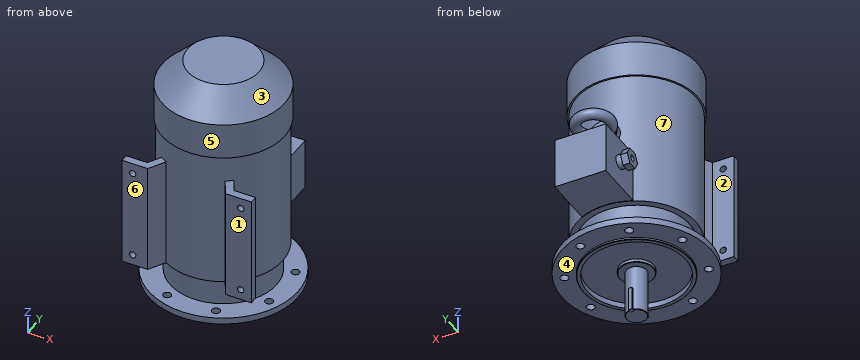
from build123d import *

# Parameters (mm, degrees)
SKETCH_1_R           = 24
EXTRUDE_1_DEPTH      = 110
SKETCH_2_W           = 9
SKETCH_2_H           = 9
EXTRUDE_2_DEPTH      = 0.1
EXTRUDE_2_DEPTH_BACK = 55
SKETCH_3_R           = 175
EXTRUDE_3_DEPTH      = 15
SKETCH_4_R           = 125
SKETCH_4_R_2         = 116
EXTRUDE_4_DEPTH      = 5
SKETCH_5_R           = 116
SKETCH_5_R_2         = 40
CUT_EXTRUDE_1_DEPTH  = 8
CHAMFER_1_SIZE       = 1
SKETCH_6_R           = 9.5
CUT_EXTRUDE_2_DEPTH  = 16
SKETCH_7_R           = 125
EXTRUDE_5_DEPTH      = 68
SKETCH_8_R           = 140
EXTRUDE_6_DEPTH      = 322
SKETCH_9_R           = 144
EXTRUDE_7_DEPTH      = 145
CHAMFER_2_SIZE       = 60
EXTRUDE_8_DEPTH      = 260
CUT_EXTRUDE_3_REACH  = 337
SKETCH_11_R          = 7.5
SKETCH_12_W          = 120
SKETCH_12_H          = 120
EXTRUDE_9_DEPTH      = 245
SKETCH_13_R          = 35
EXTRUDE_10_DEPTH     = 150
CHAMFER_3_SIZE       = 1
SKETCH_15_R          = 12
SKETCH_16_R          = 16
EXTRUDE_11_DEPTH     = 14
EXTRUDE_12_DEPTH     = 16
SKETCH_18_R          = 7
CUT_EXTRUDE_4_DEPTH  = 16


with BuildPart() as part:
    # Эскиз1 → Вытянуть1 (new body)
    with BuildSketch(Plane.XY):
        Circle(SKETCH_1_R)
    extrude(amount=EXTRUDE_1_DEPTH)

    # Эскиз2 → Вытянуть2 (add, two sides)
    with BuildSketch(Plane(origin=(0, 0, 0), x_dir=(-1, 0, 0), z_dir=(0, 0, -1))) as extrude_2_sk:
        with Locations((0, 23)):
            Rectangle(SKETCH_2_W, SKETCH_2_H)
    extrude(amount=EXTRUDE_2_DEPTH)
    extrude(extrude_2_sk.sketch, amount=-EXTRUDE_2_DEPTH_BACK)

    # Эскиз3 → Вытянуть3 (add)
    with BuildSketch(Plane.XY.offset(110)):
        Circle(SKETCH_3_R)
    extrude(amount=EXTRUDE_3_DEPTH)

    # Эскиз4 → Вытянуть4 (add)
    with BuildSketch(Plane(origin=(0, 0, 110), x_dir=(-1, 0, 0), z_dir=(0, 0, -1))):
        with Locations(Location((0, 0, 0), (0, 0, 180))):  # turned: the seam where the file's is
            Circle(SKETCH_4_R)
        Circle(SKETCH_4_R_2, mode=Mode.SUBTRACT)
    extrude(amount=EXTRUDE_4_DEPTH)

    # Эскиз5 → Вырез-Вытянуть1 (cut)
    with BuildSketch(Plane(origin=(0, 0, 110), x_dir=(-1, 0, 0), z_dir=(0, 0, -1))):
        Circle(SKETCH_5_R)
        Circle(SKETCH_5_R_2, mode=Mode.SUBTRACT)
    extrude(amount=-CUT_EXTRUDE_1_DEPTH, mode=Mode.SUBTRACT)

    # Фаска1
    chamfer_1_edges = [part.edges().sort_by_distance(p)[0] for p in [
        (-125, 0, 105),
        (40, 0, 110),
        (-15.297058541, -18.493242009, 0),
    ]]
    chamfer(chamfer_1_edges, length=CHAMFER_1_SIZE)

    # Эскиз6 → Вырез-Вытянуть2 (cut, through all)
    with BuildSketch(Plane(origin=(0, 0, 110), x_dir=(-1, 0, 0), z_dir=(0, 0, -1))):
        with Locations((-57.402514855, 138.581929877)):
            Circle(SKETCH_6_R)
        with Locations((57.402514855, 138.581929877)):
            Circle(SKETCH_6_R)
        with Locations((138.581929877, 57.402514855)):
            Circle(SKETCH_6_R)
        with Locations((138.581929877, -57.402514855)):
            Circle(SKETCH_6_R)
        with Locations((57.402514855, -138.581929877)):
            Circle(SKETCH_6_R)
        with Locations((-57.402514855, -138.581929877)):
            Circle(SKETCH_6_R)
        with Locations((-138.581929877, -57.402514855)):
            Circle(SKETCH_6_R)
        with Locations((-138.581929877, 57.402514855)):
            Circle(SKETCH_6_R)
    extrude(amount=-CUT_EXTRUDE_2_DEPTH, mode=Mode.SUBTRACT)

    # Эскиз7 → Вытянуть5 (add)
    with BuildSketch(Plane.XY.offset(125)):
        Circle(SKETCH_7_R)
    extrude(amount=EXTRUDE_5_DEPTH)

    # Эскиз8 → Вытянуть6 (add)
    with BuildSketch(Plane.XY.offset(193)):
        Circle(SKETCH_8_R)
    extrude(amount=EXTRUDE_6_DEPTH)

    # Эскиз9 → Вытянуть7 (add)
    with BuildSketch(Plane.XY.offset(515)):
        Circle(SKETCH_9_R)
    extrude(amount=EXTRUDE_7_DEPTH)

    # Фаска2
    chamfer_2_edges = [part.edges().sort_by_distance(p)[0] for p in [
        (-144, 0, 660),
    ]]
    chamfer(chamfer_2_edges, length=CHAMFER_2_SIZE)

    # Эскиз10 → Вытянуть8 (add)
    with BuildSketch(Plane(origin=(0, 0, 193), x_dir=(-1, 0, 0), z_dir=(0, 0, -1))):
        Polygon((-152, -160), (-91.607695155, -160), (-51.945448858, -91.302974272), (-67.533906126, -82.302974272), (-102, -142), (-152, -142), align=None)
        Polygon((91.607695155, -160), (51.945448858, -91.302974272), (67.533906126, -82.302974272), (102, -142), (152, -142), (152, -160), align=None)
    extrude(amount=-EXTRUDE_8_DEPTH)

    # Эскиз11 → Вырез-Вытянуть3 (cut, up to next)
    with BuildSketch(Plane.XZ.offset(160), mode=Mode.PRIVATE) as cut_extrude_3_sk1:
        with Locations((-127, 218)):
            Circle(SKETCH_11_R)
    cut_extrude_3_tool1 = extrude(cut_extrude_3_sk1.sketch, amount=-CUT_EXTRUDE_3_REACH, mode=Mode.PRIVATE) & part.part
    add(cut_extrude_3_tool1.solids().sort_by_distance((-127, -160, 218))[0], mode=Mode.SUBTRACT)
    # Эскиз11 → Вырез-Вытянуть3 (cut, up to next)
    with BuildSketch(Plane.XZ.offset(160), mode=Mode.PRIVATE) as cut_extrude_3_sk2:
        with Locations((127, 218)):
            Circle(SKETCH_11_R)
    cut_extrude_3_tool2 = extrude(cut_extrude_3_sk2.sketch, amount=-CUT_EXTRUDE_3_REACH, mode=Mode.PRIVATE) & part.part
    add(cut_extrude_3_tool2.solids().sort_by_distance((127, -160, 218))[0], mode=Mode.SUBTRACT)
    # Эскиз11 → Вырез-Вытянуть3 (cut, up to next)
    with BuildSketch(Plane.XZ.offset(160), mode=Mode.PRIVATE) as cut_extrude_3_sk3:
        with Locations((-127, 428)):
            Circle(SKETCH_11_R)
    cut_extrude_3_tool3 = extrude(cut_extrude_3_sk3.sketch, amount=-CUT_EXTRUDE_3_REACH, mode=Mode.PRIVATE) & part.part
    add(cut_extrude_3_tool3.solids().sort_by_distance((-127, -160, 428))[0], mode=Mode.SUBTRACT)
    # Эскиз11 → Вырез-Вытянуть3 (cut, up to next)
    with BuildSketch(Plane.XZ.offset(160), mode=Mode.PRIVATE) as cut_extrude_3_sk4:
        with Locations((127, 428)):
            Circle(SKETCH_11_R)
    cut_extrude_3_tool4 = extrude(cut_extrude_3_sk4.sketch, amount=-CUT_EXTRUDE_3_REACH, mode=Mode.PRIVATE) & part.part
    add(cut_extrude_3_tool4.solids().sort_by_distance((127, -160, 428))[0], mode=Mode.SUBTRACT)

    # Эскиз12 → Вытянуть9 (add)
    with BuildSketch(Plane(origin=(0, 0, 0), x_dir=(1, 0, 0), z_dir=(0, 1, 0))):
        with Locations((0, -254)):
            Rectangle(SKETCH_12_W, SKETCH_12_H)
    extrude(amount=EXTRUDE_9_DEPTH)

    # Эскиз13 → Вытянуть10 (add)
    with BuildSketch(Plane(origin=(0, 0, 0), x_dir=(1, 0, 0), z_dir=(0, 1, 0))):
        with Locations(Location((0, -371, 0), (0, 0, 90))):  # turned: the seam where the file's is
            Circle(SKETCH_13_R)
    extrude(amount=EXTRUDE_10_DEPTH)

    # Фаска3
    chamfer_3_edges = [part.edges().sort_by_distance(p)[0] for p in [
        (0, 150, 406),
    ]]
    chamfer(chamfer_3_edges, length=CHAMFER_3_SIZE)

    # По траектории1: sweep along a path in Эскиз14
    with BuildLine(Plane.XY.offset(370)) as sweep_1_path:
        CenterArc((0, 188), 38, 0, 360)
    # Эскиз15 → По траектории1 (sweep)
    with BuildSketch(Plane(origin=(0, 0, 0), x_dir=(0, 0, -1), z_dir=(1, 0, 0))):
        with Locations((-370, 226)):
            Circle(SKETCH_15_R)
    sweep(path=sweep_1_path.line)

    # Эскиз16 → Вытянуть11 (add)
    with BuildSketch(Plane.ZY.offset(60)):
        with Locations(Location((254, 185, 0), (0, 0, 180))):  # turned: the seam where the file's is
            Circle(SKETCH_16_R)
    extrude(amount=EXTRUDE_11_DEPTH)

    # Эскиз17 → Вытянуть12 (add)
    with BuildSketch(Plane.ZY.offset(74)):
        Polygon((254, 207.516660498), (234.5, 196.258330249), (234.5, 173.741669751), (254, 162.483339502), (273.5, 173.741669751), (273.5, 196.258330249), align=None)
    extrude(amount=EXTRUDE_12_DEPTH)

    # Эскиз18 → Вырез-Вытянуть4 (cut)
    with BuildSketch(Plane.ZY.offset(90)):
        with Locations((254, 185)):
            Circle(SKETCH_18_R)
    extrude(amount=-CUT_EXTRUDE_4_DEPTH, mode=Mode.SUBTRACT)


solid = part.part
Work out the finished part from the listing and answer in its coordinate system (mm). Face numbers are marked on the shaded views. A direction names the side the tool comes from. Round coordinates to 2 decimals unless told otherwise and drop trailing zeros. Write each loop counter-clockwise with the first axis right and the second up, starting at its lowest first coordinate (ties: lowest second). Pieces come first, ordered by that corner, then holes.
1) A tool of negligible diameter and unlimited length cuts with its end or side. For the marked faces 4, 5, 6 and 7, from which of +Z, -Z, +X, -X, +Y, -Y can it reach the whole face along a straight path? Write none if from no direction.
2) A cutting plane is placed at D-D (z = 82). Give the vertices of the cut face in (x, y), plus the area to 3 significant figures.
3) Straight lines are drawn through the part: line 1 (X direction, y = 197, z = 204); line 2 (Z direction, x = 63, y = 46.5); line 3 (X direction, y = 63.5, z = 526.5). For each, find the intervals that lie inside material, in ascending order.
4) A cutting plane is placed at B-B (z = 371). Give the vertices of the cut face in (x, y), plus the area to 3 significant figures.
5) A cutting plane is placed at A-A (z = 218). Give the vertices of the cut face in (x, y), plus the area to 3 significant figures.
6) A cutting plane is placed at C-C (z = 557). Give the vertices of the cut face in (x, y).
7) Given pin 1 Ø2 at (x, y) = (98, -105.5) entering from -Z; pin 2 Ø17 at (x, y) = (57.4, -138.58) entering from -Z; pin 3 Ø15 at (x, y) = (-57.4, 138.58) entering from +Z, each flat-ended and moving along its own axis, determine where each tip first touches the part or whether it passes through.
8) The mould has two halves that part along Y. Classify the marked faces 1, 2 and 3: pulls with the +Y half, pulls with the -Y half, needs draft (parallel to the pull), parting line crosses it, or undercut.
Completed:
1. face 4: -Z
1. face 5: +Z
1. face 6: +Z, -Z, +X, -X, -Y
1. face 7: none
2. outline: circle Ø48 at (0, 0)
2. area: 1,810 mm2
3. line 1: x = -60 to 60
3. line 2: z = 118 to 660
3. line 3: x = -129.24 to 129.24
4. outline: (-152, -160) - (-91.61, -160) - (-69.42, -121.57) arc R140 ccw to (69.42, -121.57) - (91.61, -160) - (152, -160) - (152, -142) - (102, -142) - (84.47, -111.64) arc R140 ccw to (35, 135.55) - (35, 149) - (34, 150) - (32.43, 150) arc R49.96 ccw (long way) to (-32.43, 150) - (-34, 150) - (-35, 149) - (-35, 135.55) arc R140 ccw to (-84.47, -111.64) - (-102, -142) - (-152, -142) - close; hole circle Ø52.08 at (0, 188)
4. area: 71,000 mm2
5. outline: (-152, -160) - (-134.5, -160) - (-134.5, -142) - (-152, -142) - close; (-119.5, -160) - (-91.61, -160) - (-69.42, -121.57) arc R140 ccw to (69.42, -121.57) - (91.61, -160) - (119.5, -160) - (119.5, -142) - (102, -142) - (84.47, -111.64) arc R140 ccw to (60, 126.49) - (60, 245) - (-60, 245) - (-60, 126.49) arc R140 ccw to (-84.47, -111.64) - (-102, -142) - (-119.5, -142) - close; (134.5, -160) - (152, -160) - (152, -142) - (134.5, -142) - close
5. area: 77,600 mm2
6. outline: circle Ø288 at (0, 0)
7. pin 1: stops at z = 110
7. pin 2: stops at z = 515
7. pin 3: stops at z = 601.5
8. face 1: pulls with the -Y half
8. face 2: undercut
8. face 3: parting line crosses it
